Design review of the part shown in the three views and the two pictorial views. Dimensions are in mm from the part's minimum x, y and z. Give positions to 0.01 mm unless a question says otherwise; leave off trailing zeros. Loops run counter-clockwise (first coordinate to the right, second up) from the corner with the lowest first, then second, coordinate; pieces in that order, holes last. Notation, with made-up numbers: (-20.5, 60.5) - (18.5, 60.5) arc R26 cw to (18.5, 79.5) - close; hole circle Ø2 at (68, -24.5). An arc over 180 degrees is marked (long way). Answer as a JSON object with one key per item and string values.
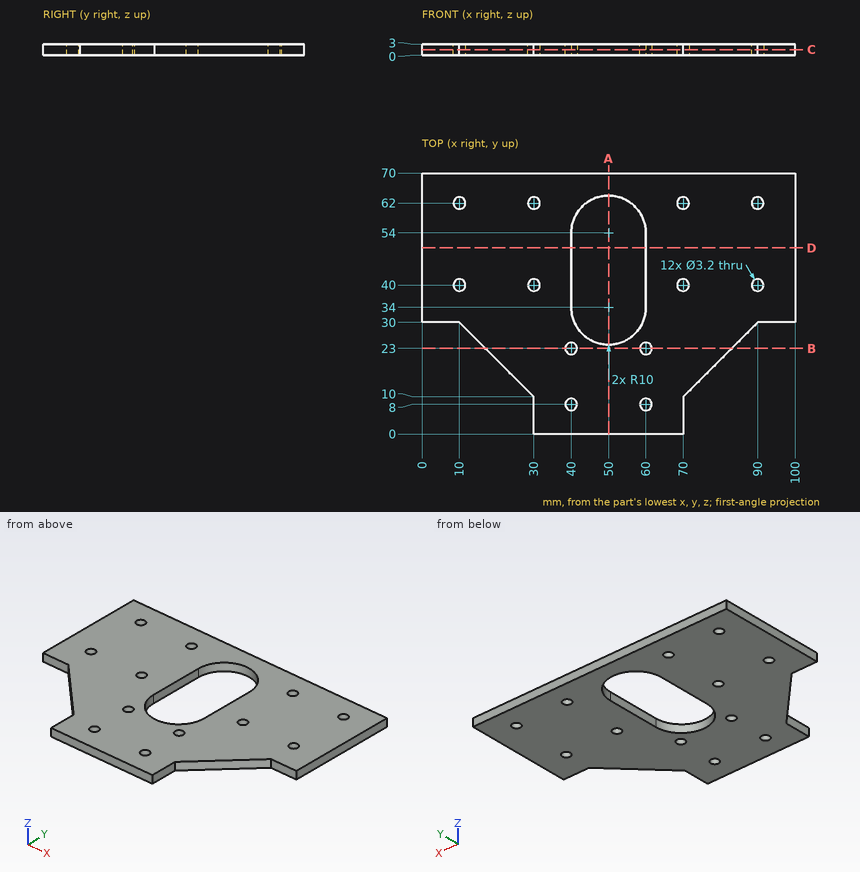
Q1. Clearance check with flat-ended pins moving along their axes: pin 1 Ø1.5 at (x, z) = (5.5, 2) entering from -Y; pin 2 Ø0.9 at (y, z) = (4.5, 1.5) entering from -X; pin 3 Ø1.9 at (x, y) = (60, 8) entering from +Z. State where each tip first meets the part, or that it passes through.
Results:
{"pin 1": "stops at y = 30", "pin 2": "stops at x = 30", "pin 3": "passes through"}
Q2. Consider section A-A, the plane x = 50. State the section outline as (y, z) points, plus the area to 3 significant figures.
Results:
{"outline": "(0, 0) - (24, 0) - (24, 3) - (0, 3) - close; (64, 0) - (70, 0) - (70, 3) - (64, 3) - close", "area": "90.0 mm^2"}
Q3. To check wall thickness, follow probe 1 along Y at (x, z) = (10, 0.7); probe 2 along X at (y, z) = (37.5, 2.55); probe 3 along X at (y, z) = (39, 1.55). State the ranges of each line that lie inside material, in increasing order. Write a range as [from, to].
Results:
{"probe 1": "y = [30, 38.4], [41.6, 60.4], [63.6, 70]", "probe 2": "x = [0, 40], [60, 100]", "probe 3": "x = [0, 8.75], [11.25, 28.75], [31.25, 40], [60, 68.75], [71.25, 88.75], [91.25, 100]"}
Q4. Consider section B-B, the plane y = 23. State the section outline as (x, z) points.
Results:
{"outline": "(17, 0) - (38.4, 0) - (38.4, 3) - (17, 3) - close; (41.6, 0) - (58.4, 0) - (58.4, 3) - (41.6, 3) - close; (61.6, 0) - (83, 0) - (83, 3) - (61.6, 3) - close"}
Q5. Consider section C-C, the plane z = 1.5. State how many separate pieces and enclosed holes the cut face has, plus the area to 3 significant figures.
Results:
{"separate pieces": "1", "enclosed holes": "13", "area": "4,790 mm^2"}
Q6. Consider section D-D, the plane y = 50. State the section outline as (x, z) points, plus the area to 3 significant figures.
Results:
{"outline": "(0, 0) - (40, 0) - (40, 3) - (0, 3) - close; (60, 0) - (100, 0) - (100, 3) - (60, 3) - close", "area": "240 mm^2"}
